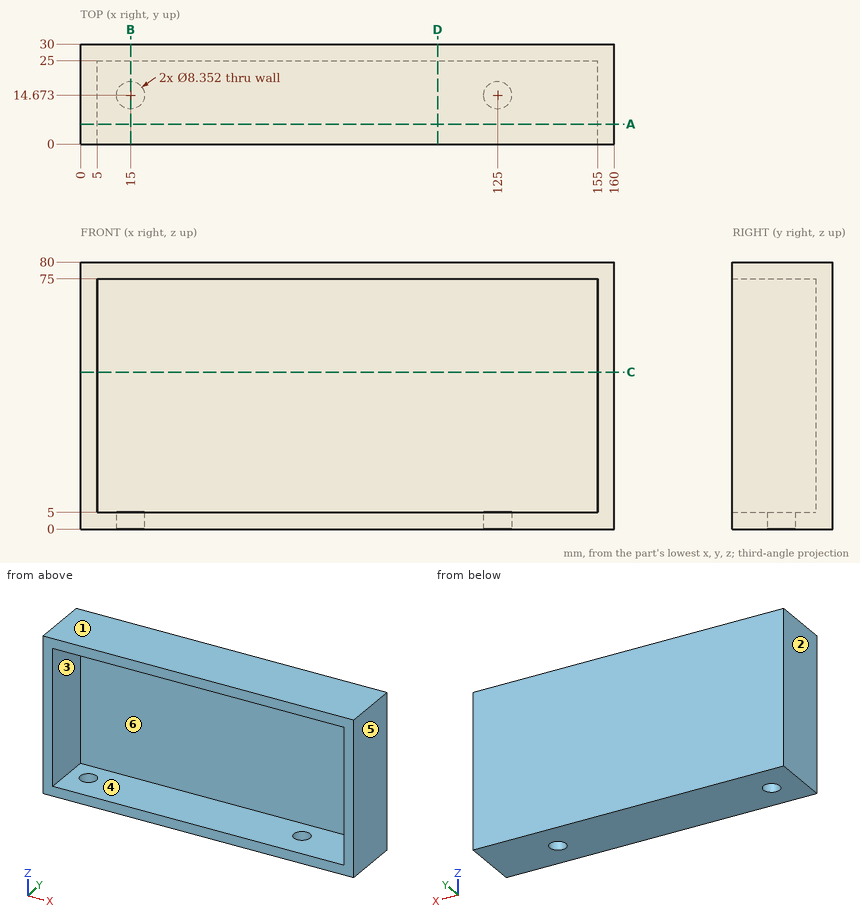
Input: dimensioned drawing with shaded views. Units: mm. Origin: part minimum x, y, z. A direction names the side the tool comes from. Give positions to 0.01 mm unless a question says otherwise; leave off trailing zeros. Write each loop counter-clockwise with the first axis right and the second up, starting at its lowest first coordinate (ties: lowest second). Pieces come first, ordered by that corner, then holes.
Q1. First-contact query: P1, Ø12.5, axis at x = 110, y = 16, coming from the -Z side; P2, Ø5, axis at x = 109.5, z = 49, coming from the -Y side. Flat tips, straight axial feed; report the tip coordinate or a pass-through.
Q2. Pull-direction query (Z, two-part tool) for the marked faces 1, 2, 3 and 4; classes: pulls with the +Z half, pulls with the -Z half, needs draft (parallel to the pull), parting line crosses it, or undercut.
Q3. Section A-A, the plane y = 6. Output: boundary loops of the cut face in (x, z), plus the area to 3 significant figures.
Q4. Section B-B, the plane x = 15. Output: boundary loops of the cut face in (y, z).
Q5. Material intervals for probe 1 along Z at (x, y) = (47.5, 7.5); probe 2 along X at (y, z) = (21.5, 32.5); probe 3 along Y at (x, z) = (15, 1.7), sorted ascending.
Q6. Set-up query: the marked faces 5 and 6. Return all of +Z, -Z, +X, -X, +Y, -Y with unobstructed straight access to the full face (end or side cutting, diameter ignored); none if empty.
Q7. Section C-C, the plane z = 47. Output: boundary loops of the cut face in (x, y), plus the area to 3 significant figures.
Q8. Section D-D, the plane x = 107. Output: boundary loops of the cut face in (y, z), plus the area to 3 significant figures.
Filled in:
1. P1: stops at z = 0
1. P2: stops at y = 25
2. face 1: pulls with the +Z half
2. face 2: needs draft
2. face 3: undercut
2. face 4: undercut
3. outline: (0, 0) - (160, 0) - (160, 80) - (0, 80) - close; hole (5, 5) - (155, 5) - (155, 75) - (5, 75) - close
3. area: 2,300 mm2
4. outline: (0, 0) - (10.5, 0) - (10.5, 5) - (0, 5) - close; (0, 75) - (25, 75) - (25, 5) - (18.85, 5) - (18.85, 0) - (30, 0) - (30, 80) - (0, 80) - close
5. probe 1: z = 0 to 5, 75 to 80
5. probe 2: x = 0 to 5, 155 to 160
5. probe 3: y = 0 to 10.5, 18.85 to 30
6. face 5: +Z, -Z, +X, +Y, -Y
6. face 6: -Y
7. outline: (0, 0) - (5, 0) - (5, 25) - (155, 25) - (155, 0) - (160, 0) - (160, 30) - (0, 30) - close
7. area: 1,050 mm2
8. outline: (0, 0) - (30, 0) - (30, 80) - (0, 80) - (0, 75) - (25, 75) - (25, 5) - (0, 5) - close
8. area: 650 mm2
